Answer from the drawing. Dimensions are ordinates in mm from the lowest x, y and z of the part. Coordinates: 2 decimals unless noted, no trailing zeros. Write each loop counter-clockwise with the first axis right and the second up, starting at its lowest first coordinate (ties: lowest second). Pieces come first, ordered by that corner, then holes. Notation, with made-up numbers: (10, 10) -> (50, 10) arc R25 cw to (50, 29) -> close; hole circle Ø10 at (4.5, -38). An arc over 180 degrees is marked (long way). Use CSV: the item, a comma, the result in double quotes.
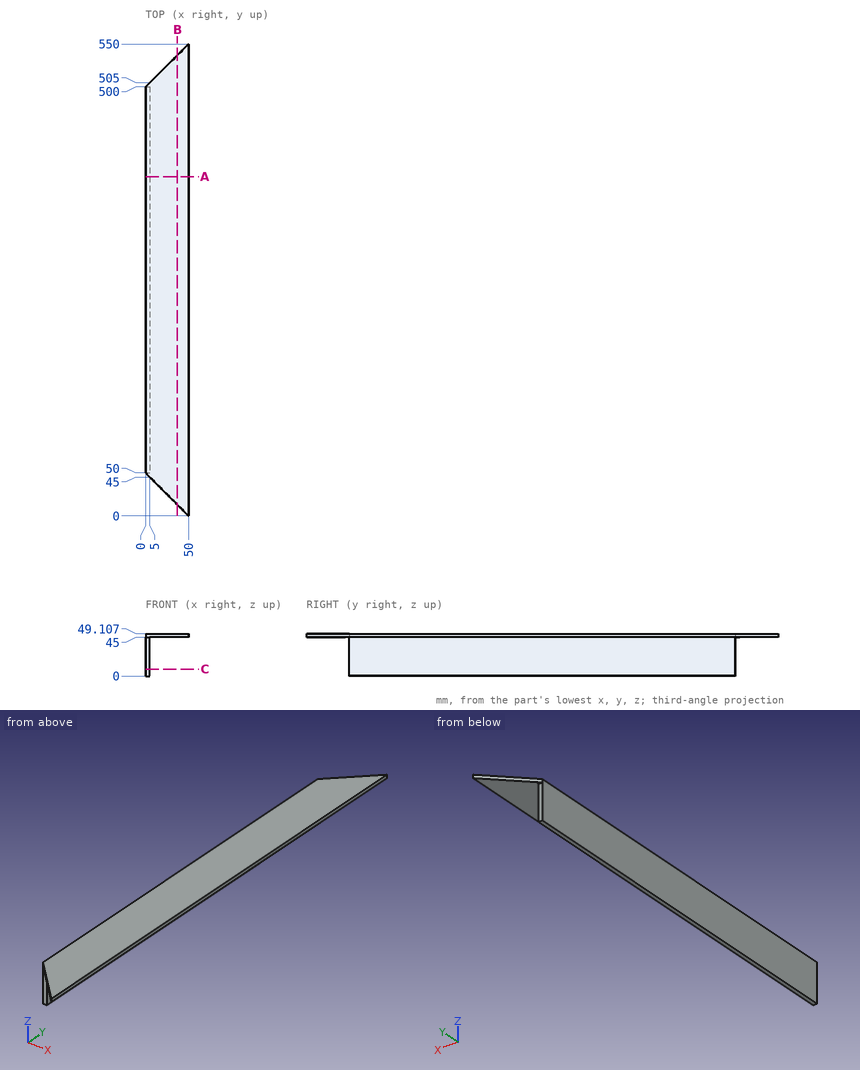
1. A cutting plane is placed at A-A (y = 395.5). Give the vertices of the cut face in (x, z).
Solutions:
outline,"(0, 0) -> (5, 0) -> (5, 45) -> (50, 45) -> (50, 49.11) -> (0, 49.11) -> close"
2. Each of these flat-tipped pins is pushed along its axis until it touches: pin 1 Ø22.5 at (y, z) = (163, 22) entering from +X; pin 2 Ø12 at (x, y) = (21.5, 448.5) entering from -Z; pin 3 Ø4 at (x, z) = (3.5, 15.5) entering from -Y; pin 4 Ø5 at (y, z) = (67, 35) entering from -X. Where does it stop, or does it pass through?
Solutions:
pin 1,"stops at x = 5"
pin 2,"stops at z = 45"
pin 3,"stops at y = 50"
pin 4,"stops at x = 0"
3. A cutting plane is placed at B-B (x = 37). Give the vertices of the cut face in (y, z).
Solutions:
outline,"(13, 45) -> (537, 45) -> (537, 49.11) -> (13, 49.11) -> close"
4. Find the intervals of material crossed by line 1 along Z through (x, y) = (11.5, 198.5); line 2 along X through (y, z) = (238.5, 37); line 3 along Y through (x, z) = (3.5, 10), in increasing order.
Solutions:
line 1,"z = 45 to 49.11"
line 2,"x = 0 to 5"
line 3,"y = 50 to 500"
5. A cutting plane is placed at C-C (z = 8). Give the vertices of the cut face in (x, y), and give its area (3 significant figures).
Solutions:
outline,"(0, 50) -> (5, 50) -> (5, 500) -> (0, 500) -> close"
area,"2,250 mm^2"
